from build123d import *

# Parameters (mm, degrees)
F0_W           = 150
F0_H           = 50
F1_DEPTH       = 15
F3_D           = 7
F3_CBORE_D     = 11.1
F3_CBORE_DEPTH = 7
F4_D           = 6
F5_D           = 8
F6_D           = 16.5


with BuildPart() as f1:
    # F0 (on Top) → F1 (new body)
    with BuildSketch(Plane.XY):
        with Locations((75, 25)):
            Rectangle(F0_W, F0_H)
    extrude(amount=-F1_DEPTH)

    # F3 (through all)
    with Locations(Plane.XY):
        with Locations((10, 25), (140, 25)):
            CounterBoreHole(F3_D / 2, F3_CBORE_D / 2, F3_CBORE_DEPTH)

    # F4 (through all)
    with Locations(Plane.XY):
        with Locations((55, 25)):
            Hole(F4_D / 2)

    # F5 (through all)
    with Locations(Plane.XY):
        with Locations((75, 25)):
            Hole(F5_D / 2)

    # F6 (through all)
    with Locations(Plane.XY):
        with Locations((100, 25)):
            Hole(F6_D / 2)


solid = f1.part
Could you check a few things on this model? Use its own coordinates, in mm. A direction names the side the tool comes from. Give positions to 0.01 mm unless a question says otherwise; leave off trailing zeros. Order: outer loops, then holes, each group sorted by start corner. A loop starts at its lowest first (then second) coordinate and runs counter-clockwise, first axis right, second up. Notation, with made-up numbers: (34.5, 36.25) -> (75.5, 36.25) arc R20 ccw to (75.5, 56.25) -> close; hole circle Ø7 at (87.25, 18). An arc over 180 degrees is marked (long way). Answer in a Markdown table with one row per item. Add a question column.
Item 1: Imagine slicing it at A-A (x = 10). List the corners of the cut face in (y, z) for me.
Item 2: Imagine slicing it at B-B (y = 25). Count the separate pieces of the cut face and the enclosed holes in it, and give its area (3 significant figures).
Item 3: Please list where these lines run through material, in increasing order: probe 1 along Y at (x, z) = (55, -4); probe 2 along X at (y, z) = (27.5, -10.25); probe 3 along Y at (x, z) = (75, -4.5).
Item 4: Imagine slicing it at C-C (z = -5). List the corners of the cut face in (x, y) for me.
Item 5: We'd pull the mould along Y, two halves only. Please class faces 3 (the flat face through (14, 25, -7)), 4 (the flat face through (74, 31, 0)), 5 (the flat face through (74, 50, -7)): pulls with the +Y half, pulls with the -Y half, needs draft (parallel to the pull), parting line crosses it, or undercut.
Item 6: I'm going to push flat-ended pins straight in: P1, Ø9, axis at x = 10, y = 25, coming from the -Z side; P2, Ø6.5, axis at x = 140, y = 25, coming from the +Z side. Where does each tip first touch, or does it pass through?
Item 7: Imagine slicing it at D-D (x = 75). List the corners of the cut face in (y, z) for me.
Item 8: For faces 1 (the flat face through (144, 25, -7)), 2 (the cylindrical face through (136.66, 26.05, -11.06)), which set-ups out of +Z, -Z, +X, -X, +Y, -Y let a thin tool reach every point of the face, with its end or its side?
Result:
| question | item | result |
|---|---|---|
| 1 | outline | (0, -15) -> (21.5, -15) -> (21.5, -7) -> (19.45, -7) -> (19.45, 0) -> (0, 0) -> close; (28.5, -15) -> (50, -15) -> (50, 0) -> (30.55, 0) -> (30.55, -7) -> (28.5, -7) -> close |
| 2 | separate pieces | 6 |
| 2 | enclosed holes | 0 |
| 2 | area | 1,530 mm2 |
| 3 | probe 1 | 0 to 22, 28 to 50 |
| 3 | probe 2 | 0 to 7.55, 12.45 to 53.34, 56.66 to 71.88, 78.12 to 92.14, 107.86 to 137.55, 142.45 to 150 |
| 3 | probe 3 | 0 to 21, 29 to 50 |
| 4 | outline | (0, 0) -> (150, 0) -> (150, 50) -> (0, 50) -> close; hole circle Ø11.1 at (10, 25); hole circle Ø6 at (55, 25); hole circle Ø8 at (75, 25); hole circle Ø16.5 at (100, 25); hole circle Ø11.1 at (140, 25) |
| 5 | face 3 | undercut |
| 5 | face 4 | needs draft |
| 5 | face 5 | pulls with the +Y half |
| 6 | P1 | z = -15 |
| 6 | P2 | through |
| 7 | outline | (0, -15) -> (21, -15) -> (21, 0) -> (0, 0) -> close; (29, -15) -> (50, -15) -> (50, 0) -> (29, 0) -> close |
| 8 | face 1 | +Z |
| 8 | face 2 | +Z, -Z |
